from build123d import *

# Parameters (mm, degrees)
SKETCH1_W           = 1
SKETCH1_H           = 35
SHELL1_T            = -0.15
SKETCH2_W           = 6
SKETCH2_H           = 0.77
BOSS_EXTRUDE1_DEPTH = 16


with BuildPart() as part:
    # Sketch1 → Revolve1 (revolve)
    with BuildSketch(Plane.XY, mode=Mode.PRIVATE) as revolve1_sk:
        Polygon((0, 40.8), (1.585, 40.8), (3.25, 43.4), (3.25, 54), (0, 54), align=None)
        Polygon((0, 35), (1, 35), (1.585, 36.35), (1.585, 40.8), (0, 40.8), align=None)
        with Locations((0.5, 17.5)):
            Rectangle(SKETCH1_W, SKETCH1_H)
    revolve(revolve1_sk.sketch.rotate(Axis((0, 40.8, 0), (0, 1, 0)), 90), axis=Axis((0, 40.8, 0), (0, 1, 0)))

    # Shell1
    shell1_openings = [part.faces().sort_by_distance(p)[0] for p in [
        (0, 0, 0),
    ]]
    offset(amount=SHELL1_T, openings=shell1_openings, kind=Kind.INTERSECTION)

    # Sketch2 → Boss-Extrude1 (add)
    with BuildSketch(Plane(origin=(0, 54, 0), x_dir=(1, 0, 0), z_dir=(0, 1, 0))):
        Rectangle(SKETCH2_W, SKETCH2_H)
    extrude(amount=-BOSS_EXTRUDE1_DEPTH)


solid = part.part
Design review of the part built by this model. Coordinates are the model's own, in mm. A direction names the side the tool comes from. Round coordinates to 2 decimals unless told otherwise and drop trailing zeros. Order: outer loops, then holes, each group sorted by start corner. A loop starts at its lowest first (then second) coordinate and runs counter-clockwise, first axis right, second up.
1) For L1, parallel to X at y = 38.4, z = 0; L2, parallel to X at y = 41.5, z = 0.75; L3, parallel to Z at x = -0.5, y = 41 (3 decimals), list the stretches that pass through material, from the lowest coordinate up.
The answers:
L1: x = -3 to 3
L2: x = -1.89 to -1.7, 1.7 to 1.89
L3: z = -1.638 to -1.451, -0.385 to 0.385, 1.451 to 1.638
2) Clearance check with flat-ended pins moving along their axes: pin 1 Ø1.2 at (x, y) = (-2.5, 40.5) entering from +Z (3 decimals); pin 2 Ø1.6 at (x, y) = (-2.5, 40) entering from -Z (3 decimals); pin 3 Ø1.6 at (x, y) = (2, 41) entering from -Z. State where each tip first meets the part, or that it passes through.
The answers:
pin 1: stops at z = 0.385
pin 2: stops at z = -0.385
pin 3: stops at z = -1.5
3) Consider section B-B (y = 48). State the section outline as (x, z) points (3 decimals), plus the area to 3 significant figures.
The answers:
outline: circle Ø6.5 at (0, 0); (-3, -0.385) - (3, -0.385) - (3, 0.385) - (-3, 0.385) - close; hole circle Ø6.2 at (0, 0)
area: 7.61 mm2
4) Consider section A-A (x = 0). State the section outline as (y, z) points (3 decimals), plus the area to 3 significant figures.
The answers:
outline: (0, -1) - (35, -1) - (36.35, -1.585) - (40.8, -1.585) - (43.4, -3.25) - (54, -3.25) - (54, 3.25) - (43.4, 3.25) - (40.8, 1.585) - (36.35, 1.585) - (35, 1) - (0, 1) - (0, 0.85) - (35.031, 0.85) - (36.381, 1.435) - (40.844, 1.435) - (43.444, 3.1) - (53.85, 3.1) - (53.85, 0.385) - (38, 0.385) - (38, -0.385) - (53.85, -0.385) - (53.85, -3.1) - (43.444, -3.1) - (40.844, -1.435) - (36.381, -1.435) - (35.031, -0.85) - (0, -0.85) - close
area: 29.5 mm2
5) Draft analysis for pull direction Z (two halves, no side actions). For faces 4 (the flat face through (-2, 40, -0.385)), 5 (the conical face through (1.663, 41.252, -0.865)), 6 (the cylindrical face through (-0.6, 17.8, 0.6)), 7 (the flat face through (-2, 40, 0.385)), state which applies: released by +Z, released by -Z, zero draft, split by the parting line, or undercut.
The answers:
face 4: released by -Z
face 5: split by the parting line
face 6: undercut
face 7: released by +Z
6) Machinability: for faces 1 (the cylindrical face through (1.273, 38.644, -0.662)), 2 (the cylindrical face through (1, 18, 0)), 3 (the flat face through (2, 40, 0.385)), which of the approach directions +Z, -Z, +X, -X, +Y, -Y give a long, thin tool a straight path to every point of the face, cutting with its end or side? Answer none if there is none.
The answers:
face 1: none
face 2: -Y
face 3: +Z, +X, -Y
7) Consider section D-D (x = -2.25). Count the separate pieces of the cut face and the enclosed holes in it, plus the area to 3 significant figures.
The answers:
separate pieces: 1
enclosed holes: 2
area: 18.4 mm2
8) Consider section C-C (y = 32). State the section outline as (x, z) points, plus the area to 3 significant figures.
The answers:
outline: circle Ø2 at (0, 0); hole circle Ø1.7 at (0, 0)
area: 0.872 mm2
